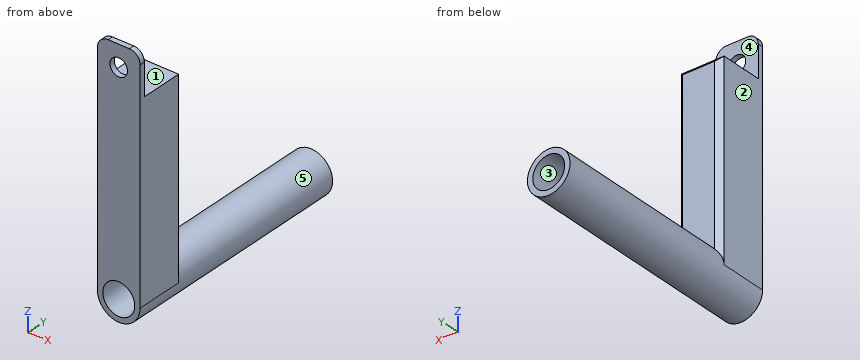
Autodesk Inventor part; units mm, degrees
ref_plane "YZ Plane" through (0, 0, 0) normal (1, 0, 0) x (0, 1, 0)
ref_plane "XZ Plane" through (0, 0, 0) normal (0, 1, 0) x (-1, 0, 0)
ref_plane "XY Plane" through (0, 0, 0) normal (0, 0, 1) x (1, 0, 0)
sketch "Sketch1" plane through (0, 0, 0) normal (0, 1, 0) x (-1, 0, 0)
  circle A0 centre (0, 0) radius 3
  circle A1 centre (0, 0) radius 4
  dimension "d0" = 6
  dimension "d1" = 8
extrude "Extrusion1" add sketch "Sketch1" along normal blind 45
sketch "Sketch2" plane through (0, 0, 0) normal (0, 1, 0) x (-1, 0, 0)
  circle A0 centre (0, 0) radius 4
  line L0 (-4, 0) -> (-4, 42)
  line L1 (-2, 44) -> (2, 44)
  line L2 (4, 42) -> (4, 0)
  arc A1 (-2, 44) -> (-4, 42) centre (-2, 42) ccw
  arc A2 (4, 42) -> (2, 44) centre (2, 42) ccw
  circle A3 centre (0, 40) radius 1.65
  point P0 (-4, 44)
  point P1 (4, 44)
  dimension "d4" = 44
  dimension "d5" = 8
  dimension "d6" = 2
  dimension "d10" = 3.3
extrude "Extrusion2" add sketch "Sketch2" along normal blind 10 contours A0 L0 A1 L1 A2 L2
chamfer "Chamfer1" distance 1 angle 45 5 edges at (4, 10, 21) (3.4142, 10, 43.4142) (0, 10, 44) (-3.4142, 10, 43.4142) (-4, 10, 21)
sketch "Sketch4" plane through (0, 10, 0) normal (0, 1, 0) x (1, 0, 0)
  circle A0 centre (0, -40) radius 1.65
  line L0 (4, -36) -> (-4, -36)
  line L1 (-4, -36) -> (-4, -44)
  line L2 (-4, -44) -> (4, -44)
  line L3 (4, -44) -> (4, -36)
  line L4 (4, -36) -> (-4, -44) construction
  line L5 (-4, -36) -> (4, -44) construction
  point P0 (0, 0)
  point P1 (-2, -44)
  point P2 (-4, -42)
extrude "Extrusion3" cut sketch "Sketch4" against normal blind 9
chamfer "Chamfer4" distance 1 angle 45 1 edges at (0, 10, 36)
properties part number "Rod Spacer" material "ABS Plastic"
Source: CAD feature listing. Evaluate the final solid. Frame: model axes, mm. Face numbers are marked on the shaded views. A direction names the side the tool comes from. Give positions to 0.01 mm unless a question says otherwise; leave off trailing zeros. Loops run counter-clockwise (first coordinate to the right, second up) from the corner with the lowest first, then second, coordinate; pieces in that order, holes last. Notation, with made-up numbers: (-33.75, 59.5) -> (15.25, 59.5) arc R33 ccw to (15.25, 97.5) -> close; hole circle Ø9 at (85.5, -40). An arc over 180 degrees is marked (long way). Use a Markdown table: item, result. Add a question column.
(1) Section query C-C (y = 14). Output: boundary loops of the cut face in (x, z), then the cut area to 3 significant figures.
(2) Section query A-A (x = 0). Output: boundary loops of the cut face in (y, z), then the cut area to 3 significant figures.
(3) Access query for the marked faces 1 and 2. Directions: +Z, -Z, +X, -X, +Y, -Y. A direction counts if a zero-diameter tool reaches every point of the face in a straight line with its end or side. Return the directions, or none.
(4) Section query D-D (z = 5). Output: boundary loops of the cut face in (x, y), then the cut area to 3 significant figures.
(5) Pull-direction query (Z, two-part tool) for the marked faces 3, 4 and 5; classes: +Z half, -Z half, draft (parallel to the pull), parting line (faces both ways), or undercut.
(6) First-contact query: pin 1 Ø4 at (x, y) = (-1, 16) entering from -Z; pin 2 Ø1.8 at (x, z) = (0.5, 22) entering from +Y. Flat tips, straight axial feed; report the tip coordinate or a pass-through.
(7) Ray query, line 1 (Z direction, x = 0, y = 0.25); line 2 (Z direction, x = 0, y = 34); line 3 (Y direction, x = -1.25, z = 5.5). Return the intervals inside material, ascending.
(8) Section query B-B (z = 40). Output: boundary loops of the cut face in (x, y), then the cut area to 3 significant figures.
Checked values:
| question | item | result |
|---|---|---|
| 1 | outline | circle Ø8 at (0, 0); hole circle Ø6 at (0, 0) |
| 1 | area | 22.0 mm^2 |
| 2 | outline | (0, -4) -> (45, -4) -> (45, -3) -> (0, -3) -> close; (0, 3) -> (45, 3) -> (45, 4) -> (10, 4) -> (10, 35) -> (9, 36) -> (1, 36) -> (1, 38.35) -> (0, 38.35) -> close; (0, 41.65) -> (1, 41.65) -> (1, 44) -> (0, 44) -> close |
| 2 | area | 414 mm^2 |
| 3 | face 1 | +Z, +X, -X, +Y |
| 3 | face 2 | +Z, -Z, -X, +Y, -Y |
| 4 | outline | (-4, 0) -> (4, 0) -> (4, 9) -> (3, 10) -> (-3, 10) -> (-4, 9) -> close |
| 4 | area | 79.0 mm^2 |
| 5 | face 3 | undercut |
| 5 | face 4 | draft |
| 5 | face 5 | parting line |
| 6 | pin 1 | z = -4 |
| 6 | pin 2 | y = 10 |
| 7 | line 1 | -4 to -3, 3 to 38.35, 41.65 to 44 |
| 7 | line 2 | -4 to -3, 3 to 4 |
| 7 | line 3 | 0 to 10 |
| 8 | outline | (-4, 0) -> (-1.65, 0) -> (-1.65, 1) -> (-4, 1) -> close; (1.65, 0) -> (4, 0) -> (4, 1) -> (1.65, 1) -> close |
| 8 | area | 4.70 mm^2 |
